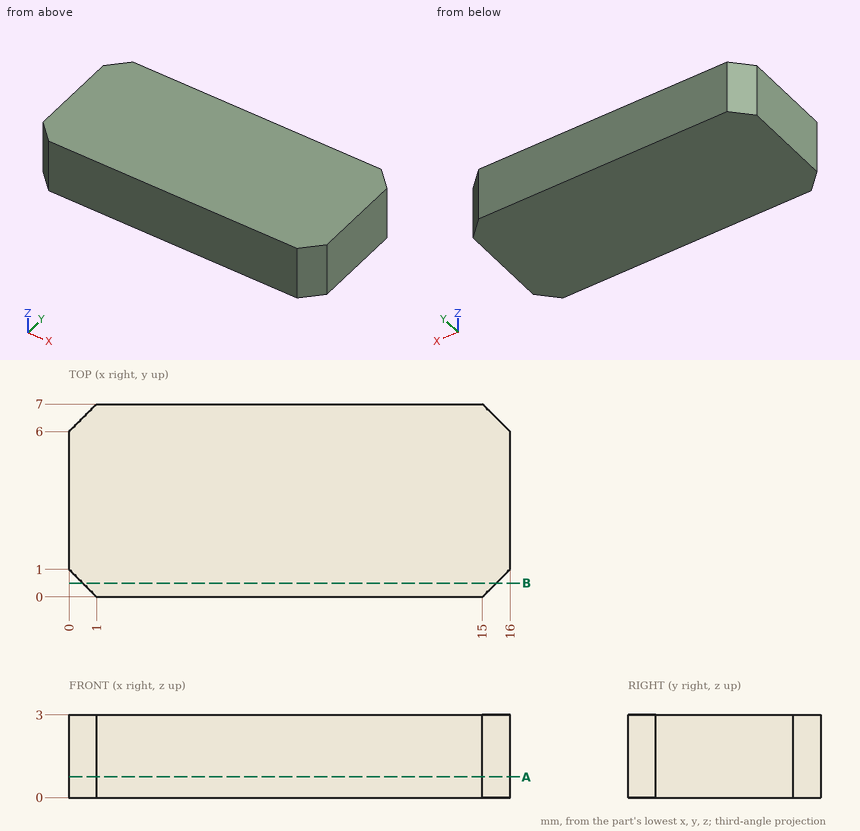
Study the drawing (mm; zero at the part's minimum x, y, z) and answer. Give positions to 0.01 mm unless a question says otherwise; leave off trailing zeros. Loops run counter-clockwise (first coordinate to the right, second up) from the corner with the lowest first, then second, coordinate; pieces in that order, holes last. Notation, with made-up numbers: (66, 5) -> (82, 5) arc R22 cw to (82, 37) -> close; hole circle Ø9 at (37.5, -37). An arc over 180 degrees is marked (long way). Use a Markdown table: item, result. Add a question column.
1) The part is cut by section B-B, the plane y = 0.5. Determine the outline of the cut face in (x, z).
2) The part is cut by section A-A, the plane z = 0.75. Determine the outline of the cut face in (x, y), plus the area to 3 significant figures.
3) Consider line 1 along X through (y, z) = (6.5, 0.7); line 2 along Y through (x, z) = (0.5, 0.85); line 3 along X through (y, z) = (6.75, 0.45). Determine where each line is inside the solid, lowest interval first.
Reported:
| question | item | result |
|---|---|---|
| 1 | outline | (0.5, 0) -> (15.5, 0) -> (15.5, 3) -> (0.5, 3) -> close |
| 2 | outline | (0, 1) -> (1, 0) -> (15, 0) -> (16, 1) -> (16, 6) -> (15, 7) -> (1, 7) -> (0, 6) -> close |
| 2 | area | 110 mm^2 |
| 3 | line 1 | x = 0.5 to 15.5 |
| 3 | line 2 | y = 0.5 to 6.5 |
| 3 | line 3 | x = 0.75 to 15.25 |
